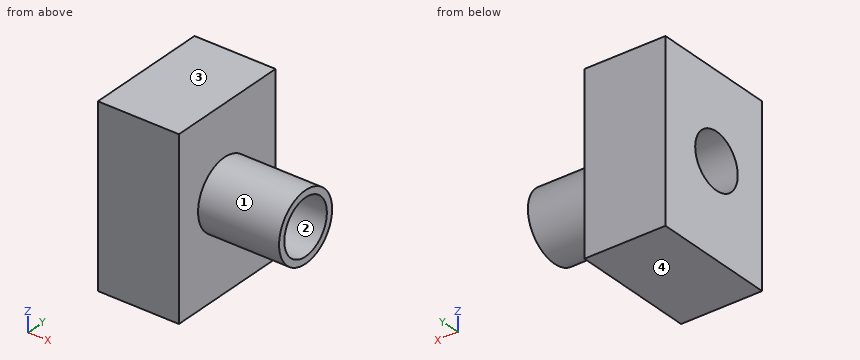
from build123d import *

# Parameters (mm, degrees)
F0_R     = 10.711856
F0_R_2   = 8.597531
F1_DEPTH = 50.8
F0_W     = 39.041024
F0_H     = 55.187622
F2_DEPTH = 25.4


with BuildPart() as f1:
    # F0 (on Right) → F1 (new body)
    with BuildSketch(Plane.YZ):
        with Locations((0, 11.128576)):
            Circle(F0_R)
        with Locations((0, 11.128576)):
            Circle(F0_R_2, mode=Mode.SUBTRACT)
    extrude(amount=F1_DEPTH)

    # F0 (on Right) → F2 (join)
    with BuildSketch(Plane.YZ):
        with Locations((1.084473, 9.880754)):
            Rectangle(F0_W, F0_H)
        with Locations((0, 11.128576)):
            Circle(F0_R, mode=Mode.SUBTRACT)
    extrude(amount=F2_DEPTH)


solid = f1.part
Source: CAD feature listing. Evaluate the final solid. Frame: model axes, mm. Face numbers are marked on the shaded views. Coordinates: 2 decimals unless noted, no trailing zeros. Loops run counter-clockwise (first coordinate to the right, second up) from the corner with the lowest first, then second, coordinate; pieces in that order, holes last. Notation, with made-up numbers: (3.5, -22) - (15.5, -22) arc R9 ccw to (15.5, -9) - close; hole circle Ø10 at (-20.5, 35). An arc over 180 degrees is marked (long way). One line per item, written item: value. Start each with the question number.
1. Section C-C (x = 23). Return the cut outline in (y, z).
2. Contact query for flat-ended pins moving along their axis: P1, Ø6, axis at y = -2.5, z = -11.5, coming from the +X side; P2, Ø15.5, axis at y = 0, z = 11.13, coming from the -X side. Output: stop coordinate, or through.
3. Mould query, pull axis Z, two halves, no side actions, for the marked faces 1, 2, 3 and 4. Classes: pulls with the +Z half, pulls with the -Z half, needs draft (parallel to the pull), parting line crosses it, or undercut.
4. Section D-D (y = -11.5). Return the cut outline in (x, z).
5. Ray query, L1, parallel to Z at x = 21, y = 0; L2, parallel to Z at x = 28, y = 0; L3, parallel to X at y = 12, z = 8.5. Return the intervals inside material, ascending.
6. Section A-A (y = 0). Return the cut outline in (x, z), and give its area (3 significant figures).
7. Section B-B (z = 13.5). Return the cut outline in (x, y), and give its area (3 significant figures).
Verdict:
1. outline: (-18.44, -17.71) - (20.6, -17.71) - (20.6, 37.47) - (-18.44, 37.47) - close; hole circle Ø17.2 at (0, 11.13)
2. P1: stops at x = 25.4
2. P2: passes through
3. face 1: parting line crosses it
3. face 2: undercut
3. face 3: pulls with the +Z half
3. face 4: pulls with the -Z half
4. outline: (0, -17.71) - (25.4, -17.71) - (25.4, 37.47) - (0, 37.47) - close
5. L1: z = -17.71 to 2.53, 19.73 to 37.47
5. L2: z = 0.42 to 2.53, 19.73 to 21.84
5. L3: x = 0 to 25.4
6. outline: (0, -17.71) - (25.4, -17.71) - (25.4, 0.42) - (50.8, 0.42) - (50.8, 2.53) - (0, 2.53) - close; (0, 19.73) - (50.8, 19.73) - (50.8, 21.84) - (25.4, 21.84) - (25.4, 37.47) - (0, 37.47) - close
6. area: 1,070 mm2
7. outline: (0, -18.44) - (25.4, -18.44) - (25.4, -10.45) - (50.8, -10.45) - (50.8, -8.26) - (0, -8.26) - close; (0, 8.26) - (50.8, 8.26) - (50.8, 10.45) - (25.4, 10.45) - (25.4, 20.6) - (0, 20.6) - close
7. area: 683 mm2
